from build123d import *

# Parameters (mm, degrees)
F0_W           = 25.4
F0_H           = 20.6375
F1_DEPTH       = 3.175
F3_D           = 3.2639
F3_CSINK_D     = 6.477
F3_CSINK_ANGLE = 82
F4_R           = 3.175


with BuildPart() as f1:
    # F0 (on Front) → F1 (new body)
    with BuildSketch(Plane.XZ):
        Rectangle(F0_W, F0_H)
    extrude(amount=F1_DEPTH)

    # F3 (through all)
    with Locations(Plane(origin=(0, 0, 0), x_dir=(-1, 0, 0), z_dir=(0, 1, 0))):
        with Locations((0, 3.96875)):
            CounterSinkHole(F3_D / 2, F3_CSINK_D / 2, counter_sink_angle=F3_CSINK_ANGLE)

    # F4
    f4_edges = [f1.edges().sort_by_distance(p)[0] for p in [
        (12.7, -1.5875, 10.31875),
        (-12.7, -1.5875, 10.31875),
        (-12.7, -1.5875, -10.31875),
        (12.7, -1.5875, -10.31875),
    ]]
    fillet(f4_edges, radius=F4_R)


solid = f1.part
Could you check a few things on this model? Use its own coordinates, in mm. Round coordinates to 2 decimals unless told otherwise and drop trailing zeros. Order: outer loops, then holes, each group sorted by start corner. A loop starts at its lowest first (then second) coordinate and runs counter-clockwise, first axis right, second up. Notation, with made-up numbers: M 9.25,7 L 34.25,7 A29 cw 34.25,38 Z; hole C 61,-39.75 d11. An arc over 180 degrees is marked long. One line per item, written item: value.
(1) Imagine slicing it at B-B (y = -2.85). Write out the boundary of the cut face in (x, z) (3 decimals).
Ans:
outline: M -12.7,-7.144 A3.175 ccw -9.525,-10.319 L 9.525,-10.319 A3.175 ccw 12.7,-7.144 L 12.7,7.144 A3.175 ccw 9.525,10.319 L -9.525,10.319 A3.175 ccw -12.7,7.144 Z; hole C 0,3.969 d3.264
(2) I need wall thicknesses on line 1 along Z through (x, y) = (0, -2.5); line 2 along Z through (x, y) = (0.5, -2.05); line 3 along X through (y, z) = (-0.55, 8.75). Which ranges of each line are inside material? Lowest first, please. Write a range as from..to.
Ans:
line 1: z = -10.32..2.34, 5.6..10.32
line 2: z = -10.32..2.42, 5.52..10.32
line 3: x = -12.26..12.26
(3) Imagine slicing it at A-A (x = 0). Write out the boundary of the cut face in (y, z) (3 decimals), and give its area (3 significant figures).
Ans:
outline: M -3.175,-10.319 L 0,-10.319 L 0,0.73 L -1.848,2.337 L -3.175,2.337 Z; M -3.175,5.601 L -1.848,5.601 L 0,7.207 L 0,10.319 L -3.175,10.319 Z
area: 52.2 mm^2
(4) If we mould it in two halves opening along Z, with no side actions, what happens to faces 1 (the flat face through (0, -2, -10.319)), 2 (the cylindrical face through (0.877, -2.521, 5.345)), 3 (the flat face through (-12.7, -2, 0))? For each: released by +Z, released by -Z, zero draft, split by the parting line, or undercut.
Ans:
face 1: released by -Z
face 2: undercut
face 3: zero draft
(5) Imagine slicing it at C-C (y = -1.25). Write out the boundary of the cut face in (x, z) (3 decimals).
Ans:
outline: M -12.7,-7.144 A3.175 ccw -9.525,-10.319 L 9.525,-10.319 A3.175 ccw 12.7,-7.144 L 12.7,7.144 A3.175 ccw 9.525,10.319 L -9.525,10.319 A3.175 ccw -12.7,7.144 Z; hole C 0,3.969 d4.304
(6) I'm going to push flat-ended pins straight in: P1, Ø10, axis at x = 6.5, z = 4.5, coming from the +Y side; P2, Ø2.5, axis at x = 0, z = 3.97, coming from the -Y side. Where does each tip first touch, or does it pass through?
Ans:
P1: stops at y = 0
P2: passes through
